from build123d import *

# Parameters (mm, degrees)
SKETCH4_R           = 100
SKETCH4_R_2         = 7.709671905
SKETCH4_R_3         = 4.293457035
SKETCH4_R_4         = 4.043319463
BOSS_EXTRUDE3_DEPTH = 0.5


with BuildPart() as part:
    # Sketch4 → Boss-Extrude3 (new body)
    with BuildSketch(Plane.XY):
        Circle(SKETCH4_R)
        with Locations((-51.833048523, 72.153357866)):
            Circle(SKETCH4_R_2, mode=Mode.SUBTRACT)
        with Locations((0.476862532, 88.839994218)):
            Circle(SKETCH4_R_2, mode=Mode.SUBTRACT)
        with Locations((52.604628307, 71.592772339)):
            Circle(SKETCH4_R_2, mode=Mode.SUBTRACT)
        with Locations((84.639214035, 26.999544775)):
            Circle(SKETCH4_R_2, mode=Mode.SUBTRACT)
        with Locations((84.344496782, -27.906591212)):
            Circle(SKETCH4_R_2, mode=Mode.SUBTRACT)
        with Locations((51.833048523, -72.153357866)):
            Circle(SKETCH4_R_2, mode=Mode.SUBTRACT)
        with Locations((-0.476862532, -88.839994218)):
            Circle(SKETCH4_R_2, mode=Mode.SUBTRACT)
        with Locations((-52.604628307, -71.592772339)):
            Circle(SKETCH4_R_2, mode=Mode.SUBTRACT)
        with Locations((-84.639214035, -26.999544775)):
            Circle(SKETCH4_R_2, mode=Mode.SUBTRACT)
        with Locations((-84.344496782, 27.906591212)):
            Circle(SKETCH4_R_2, mode=Mode.SUBTRACT)
        with Locations((-69.108190101, 58.095232128)):
            Circle(SKETCH4_R_3, mode=Mode.SUBTRACT)
        with Locations((-79.041417756, 46.2537546)):
            Circle(SKETCH4_R_4, mode=Mode.SUBTRACT)
        with Locations((-36.758575407, 83.879453202)):
            Circle(SKETCH4_R_4, mode=Mode.SUBTRACT)
        with Locations((-21.762179569, 87.620805038)):
            Circle(SKETCH4_R_3, mode=Mode.SUBTRACT)
        with Locations((19.56479337, 89.466051639)):
            Circle(SKETCH4_R_4, mode=Mode.SUBTRACT)
        with Locations((33.89624389, 83.678208545)):
            Circle(SKETCH4_R_3, mode=Mode.SUBTRACT)
        with Locations((68.415076062, 60.879659189)):
            Circle(SKETCH4_R_4, mode=Mode.SUBTRACT)
        with Locations((76.607454273, 47.773380505)):
            Circle(SKETCH4_R_3, mode=Mode.SUBTRACT)
        with Locations((91.133125041, 9.039306152)):
            Circle(SKETCH4_R_4, mode=Mode.SUBTRACT)
        with Locations((90.057220916, -6.37925513)):
            Circle(SKETCH4_R_3, mode=Mode.SUBTRACT)
        with Locations((79.041417756, -46.2537546)):
            Circle(SKETCH4_R_4, mode=Mode.SUBTRACT)
        with Locations((69.108190101, -58.095232128)):
            Circle(SKETCH4_R_3, mode=Mode.SUBTRACT)
        with Locations((36.758575407, -83.879453202)):
            Circle(SKETCH4_R_4, mode=Mode.SUBTRACT)
        with Locations((21.762179569, -87.620805038)):
            Circle(SKETCH4_R_3, mode=Mode.SUBTRACT)
        with Locations((-19.56479337, -89.466051639)):
            Circle(SKETCH4_R_4, mode=Mode.SUBTRACT)
        with Locations((-33.89624389, -83.678208545)):
            Circle(SKETCH4_R_3, mode=Mode.SUBTRACT)
        with Locations((-68.415076062, -60.879659189)):
            Circle(SKETCH4_R_4, mode=Mode.SUBTRACT)
        with Locations((-76.607454273, -47.773380505)):
            Circle(SKETCH4_R_3, mode=Mode.SUBTRACT)
        with Locations((-91.133125041, -9.039306152)):
            Circle(SKETCH4_R_4, mode=Mode.SUBTRACT)
        with Locations((-90.057220916, 6.37925513)):
            Circle(SKETCH4_R_3, mode=Mode.SUBTRACT)
        with BuildLine():
            Line((-30.083194516, -21.987342606), (-4, -37.046481981))
            ThreePointArc((-4, -37.046481981), (0, -38.118278751), (4, -37.046481981))
            Line((4, -37.046481981), (30.083194516, -21.987342606))
            ThreePointArc((30.083194516, -21.987342606), (33.011397747, -19.059139375), (34.083194516, -15.059139375))
            Line((34.083194516, -15.059139375), (34.083194516, 15.059139375))
            ThreePointArc((34.083194516, 15.059139375), (33.011397747, 19.059139375), (30.083194516, 21.987342606))
            Line((30.083194516, 21.987342606), (4, 37.046481981))
            ThreePointArc((4, 37.046481981), (0, 38.118278751), (-4, 37.046481981))
            Line((-4, 37.046481981), (-30.083194516, 21.987342606))
            ThreePointArc((-30.083194516, 21.987342606), (-33.011397747, 19.059139375), (-34.083194516, 15.059139375))
            Line((-34.083194516, 15.059139375), (-34.083194516, -15.059139375))
            ThreePointArc((-34.083194516, -15.059139375), (-33.011397747, -19.059139375), (-30.083194516, -21.987342606))
        make_face(mode=Mode.SUBTRACT)
        with BuildLine():
            ThreePointArc((-79.041417756, 9.075699852), (-78.675414747, -0.003129792), (-78.819462746, -9.088192042))
            ThreePointArc((-78.819462746, -9.088192042), (-74.705516442, -16.436532645), (-66.293727059, -16.03099205))
            ThreePointArc((-66.293727059, -16.03099205), (-58.733632242, -11.195000294), (-50.867669858, -6.874295994))
            ThreePointArc((-50.867669858, -6.874295994), (-46.483207187, 0.324262898), (-50.978822695, 7.453933594))
            ThreePointArc((-50.978822695, 7.453933594), (-58.980049319, 11.657163363), (-66.711957636, 16.33737295))
            ThreePointArc((-66.711957636, 16.33737295), (-75.12002492, 16.515457082), (-79.041417756, 9.075699852))
        make_face(mode=Mode.SUBTRACT)
        with BuildLine():
            ThreePointArc((-58.611287696, 53.801775093), (-63.651587216, 46.241716451), (-69.108190101, 38.976415985))
            ThreePointArc((-69.108190101, 38.976415985), (-70.099183862, 30.613366591), (-63.055532517, 25.99713008))
            ThreePointArc((-63.055532517, 25.99713008), (-54.096762698, 25.465817356), (-45.193419184, 24.337843877))
            ThreePointArc((-45.193419184, 24.337843877), (-37.415107618, 27.584477859), (-36.861421675, 35.994959112))
            ThreePointArc((-36.861421675, 35.994959112), (-40.86395352, 44.098446437), (-44.368240575, 52.42951721))
            ThreePointArc((-44.368240575, 52.42951721), (-51.065834671, 57.515728249), (-58.611287696, 53.801775093))
        make_face(mode=Mode.SUBTRACT)
        with BuildLine():
            ThreePointArc((-15.793637862, 77.977400904), (-24.315016806, 74.823798708), (-32.999937739, 72.153357866))
            ThreePointArc((-32.999937739, 72.153357866), (-38.717345631, 65.970000299), (-35.732267733, 58.095232128))
            ThreePointArc((-35.732267733, 58.095232128), (-28.796768484, 52.399558327), (-22.25681845, 46.2537546))
            ThreePointArc((-22.25681845, 46.2537546), (-14.055708632, 44.308359839), (-8.664210449, 50.787133672))
            ThreePointArc((-8.664210449, 50.787133672), (-7.139216391, 59.695621822), (-5.077363635, 68.49536791))
            ThreePointArc((-5.077363635, 68.49536791), (-7.506231241, 76.546946113), (-15.793637862, 77.977400904))
        make_face(mode=Mode.SUBTRACT)
        with BuildLine():
            ThreePointArc((33.05664483, 72.368309924), (24.309063587, 74.825733026), (15.713169213, 77.770169444))
            ThreePointArc((15.713169213, 77.770169444), (7.453202677, 76.128336131), (5.23950883, 68.002930089))
            ThreePointArc((5.23950883, 68.002930089), (7.502612525, 59.318449013), (9.18113045, 50.502303173))
            ThreePointArc((9.18113045, 50.502303173), (14.672493316, 44.107954347), (22.842434682, 46.180349362))
            ThreePointArc((22.842434682, 46.180349362), (29.312458747, 52.491098651), (36.152893641, 58.39831614))
            ThreePointArc((36.152893641, 58.39831614), (38.920497396, 66.339832296), (33.05664483, 72.368309924))
        make_face(mode=Mode.SUBTRACT)
        with BuildLine():
            ThreePointArc((69.280412751, 39.116984261), (63.647907924, 46.246780561), (58.424379596, 53.681419606))
            ThreePointArc((58.424379596, 53.681419606), (50.776880887, 57.208235068), (44.209971104, 51.935820089))
            ThreePointArc((44.209971104, 51.935820089), (40.936250553, 43.579708336), (37.112199574, 35.460688444))
            ThreePointArc((37.112199574, 35.460688444), (37.796301516, 27.059809469), (45.624046151, 23.934241207))
            ThreePointArc((45.624046151, 23.934241207), (54.567770937, 25.236759902), (63.573974337, 25.99509249))
            ThreePointArc((63.573974337, 25.99509249), (70.480918886, 30.793157351), (69.280412751, 39.116984261))
        make_face(mode=Mode.SUBTRACT)
        with BuildLine():
            ThreePointArc((79.041417756, -9.075699852), (78.675414747, 0.003129792), (78.819462746, 9.088192042))
            ThreePointArc((78.819462746, 9.088192042), (74.705516442, 16.436532645), (66.293727059, 16.03099205))
            ThreePointArc((66.293727059, 16.03099205), (58.733632242, 11.195000294), (50.867669858, 6.874295994))
            ThreePointArc((50.867669858, 6.874295994), (46.483207187, -0.324262898), (50.978822695, -7.453933594))
            ThreePointArc((50.978822695, -7.453933594), (58.980049319, -11.657163363), (66.711957636, -16.33737295))
            ThreePointArc((66.711957636, -16.33737295), (75.12002492, -16.515457082), (79.041417756, -9.075699852))
        make_face(mode=Mode.SUBTRACT)
        with BuildLine():
            ThreePointArc((58.611287696, -53.801775093), (63.651587216, -46.241716451), (69.108190101, -38.976415985))
            ThreePointArc((69.108190101, -38.976415985), (70.099183862, -30.613366591), (63.055532517, -25.99713008))
            ThreePointArc((63.055532517, -25.99713008), (54.096762698, -25.465817356), (45.193419184, -24.337843877))
            ThreePointArc((45.193419184, -24.337843877), (37.415107618, -27.584477859), (36.861421675, -35.994959112))
            ThreePointArc((36.861421675, -35.994959112), (40.86395352, -44.098446437), (44.368240575, -52.42951721))
            ThreePointArc((44.368240575, -52.42951721), (51.065834671, -57.515728249), (58.611287696, -53.801775093))
        make_face(mode=Mode.SUBTRACT)
        with BuildLine():
            ThreePointArc((15.793637862, -77.977400904), (24.315016806, -74.823798708), (32.999937739, -72.153357866))
            ThreePointArc((32.999937739, -72.153357866), (38.717345631, -65.970000299), (35.732267733, -58.095232128))
            ThreePointArc((35.732267733, -58.095232128), (28.796768484, -52.399558327), (22.25681845, -46.2537546))
            ThreePointArc((22.25681845, -46.2537546), (14.055708632, -44.308359839), (8.664210449, -50.787133672))
            ThreePointArc((8.664210449, -50.787133672), (7.139216391, -59.695621822), (5.077363635, -68.49536791))
            ThreePointArc((5.077363635, -68.49536791), (7.506231241, -76.546946113), (15.793637862, -77.977400904))
        make_face(mode=Mode.SUBTRACT)
        with BuildLine():
            ThreePointArc((-33.05664483, -72.368309924), (-24.309063587, -74.825733026), (-15.713169213, -77.770169444))
            ThreePointArc((-15.713169213, -77.770169444), (-7.453202677, -76.128336131), (-5.23950883, -68.002930089))
            ThreePointArc((-5.23950883, -68.002930089), (-7.502612525, -59.318449013), (-9.18113045, -50.502303173))
            ThreePointArc((-9.18113045, -50.502303173), (-14.672493316, -44.107954347), (-22.842434682, -46.180349362))
            ThreePointArc((-22.842434682, -46.180349362), (-29.312458747, -52.491098651), (-36.152893641, -58.39831614))
            ThreePointArc((-36.152893641, -58.39831614), (-38.920497396, -66.339832296), (-33.05664483, -72.368309924))
        make_face(mode=Mode.SUBTRACT)
        with BuildLine():
            ThreePointArc((-69.280412751, -39.116984261), (-63.647907924, -46.246780561), (-58.424379596, -53.681419606))
            ThreePointArc((-58.424379596, -53.681419606), (-50.776880887, -57.208235068), (-44.209971104, -51.935820089))
            ThreePointArc((-44.209971104, -51.935820089), (-40.936250553, -43.579708336), (-37.112199574, -35.460688444))
            ThreePointArc((-37.112199574, -35.460688444), (-37.796301516, -27.059809469), (-45.624046151, -23.934241207))
            ThreePointArc((-45.624046151, -23.934241207), (-54.567770937, -25.236759902), (-63.573974337, -25.99509249))
            ThreePointArc((-63.573974337, -25.99509249), (-70.480918886, -30.793157351), (-69.280412751, -39.116984261))
        make_face(mode=Mode.SUBTRACT)
    extrude(amount=BOSS_EXTRUDE3_DEPTH)


solid = part.part
Geometry: final body of the model. Coordinates: model frame, mm. Give positions to 0.01 mm unless a question says otherwise; leave off trailing zeros. Order: outer loops, then holes, each group sorted by start corner. A loop starts at its lowest first (then second) coordinate and runs counter-clockwise, first axis right, second up. Notation, with made-up numbers: (23.5, -26.75) -> (78.5, -26.75) arc R24 ccw to (78.5, -13.75) -> close; hole circle Ø10 at (6, -20). An arc over 180 degrees is marked (long way). Write each question's results on one line, items separated by ' | '.
1) Cut plane A-A (x = 0). Output: boundary loops of the cut face in (y, z).
Geometry says:
outline: (-100, 0) -> (-96.53, 0) -> (-96.53, 0.5) -> (-100, 0.5) -> close; (-81.15, 0) -> (-38.12, 0) -> (-38.12, 0.5) -> (-81.15, 0.5) -> close; (38.12, 0) -> (81.15, 0) -> (81.15, 0.5) -> (38.12, 0.5) -> close; (96.53, 0) -> (100, 0) -> (100, 0.5) -> (96.53, 0.5) -> close
2) Draft query along X for faces 1 (the face through (76.937, 27.339, 0.246)), 2 (the face through (-1, -43, 0.5)). Return one class per face: released by +X, released by -X, zero draft, split by the parting line, or undercut.
Geometry says:
face 1: undercut | face 2: zero draft
3) Line query: line 1 along Y through (x, z) = (56, 0.4); line 2 along X through (y, z) = (87.5, 0.35); line 3 along X through (y, z) = (-29, 0.05). Output: solid intervals per line, ascending.
Geometry says:
line 1: y = -82.85 to -78.64, -65.67 to -56.38, -25.63 to -10.02, 9.62 to 25.39, 56.05 to 64.67, 78.51 to 82.85 | line 2: x = -48.41 to -38.56, -34.96 to -26.05, -17.47 to -7.12, 8.07 to 16.03, 23.1 to 31.94, 35.85 to 48.41 | line 3: x = -95.7 to -92.08, -77.19 to -69.4, -36.74 to -17.94, 17.94 to 36.61, 69.1 to 76.71, 91.98 to 95.7
4) First-contact query: pin 1 Ø10.5 at (x, y) = (68.42, 60.88) entering from -Z; pin 2 Ø7.5 at (x, y) = (-19.56, -89.47) entering from -Z. Flat tips, straight axial feed; report the tip coordinate or a pass-through.
Geometry says:
pin 1: stops at z = 0 | pin 2: passes through
5) Cut plane B-B (z = 0.3). Give the number of separate pieces and of enclosed holes in the cut face, and give its area (3 significant figures).
Geometry says:
separate pieces: 1 | enclosed holes: 41 | area: 16,400 mm²
